Drawing for the job (mm, zero at the part's lowest x, y, z). Coordinates: 2 decimals unless noted, no trailing zeros. Use a Markdown table: item, result. Add a question column.
Q1. Wall check: L1, parallel to Z at x = 9.5, y = 1.8; L2, parallel to Y at x = 5, z = 2.25 (1 decimal); L3, parallel to Z at x = 15.25, y = 2.8. Give the ranges that are in metal, low to high. Write a range as from..to.
Q2. Slice it at A-A on x = 9.5. Count the separate pieces of the cut face and the enclosed holes in it.
Q3. Pin check, flat tips, straight feed: pin 1 Ø3 at (x, z) = (15.35, 9.5) entering from +Y (1 decimal); pin 2 Ø4.5 at (x, z) = (3.65, 9.5) entering from +Y; pin 3 Ø1 at (x, y) = (4, 1) entering from -Z; pin 4 Ø1 at (x, y) = (8, 0.5) entering from -Z. Stop position of each tip, or through.
Q4. Mould opens along Y. For the marked faces 1, 2 and 3 say: released by +Y, released by -Y, zero draft, split by the parting line, or undercut.
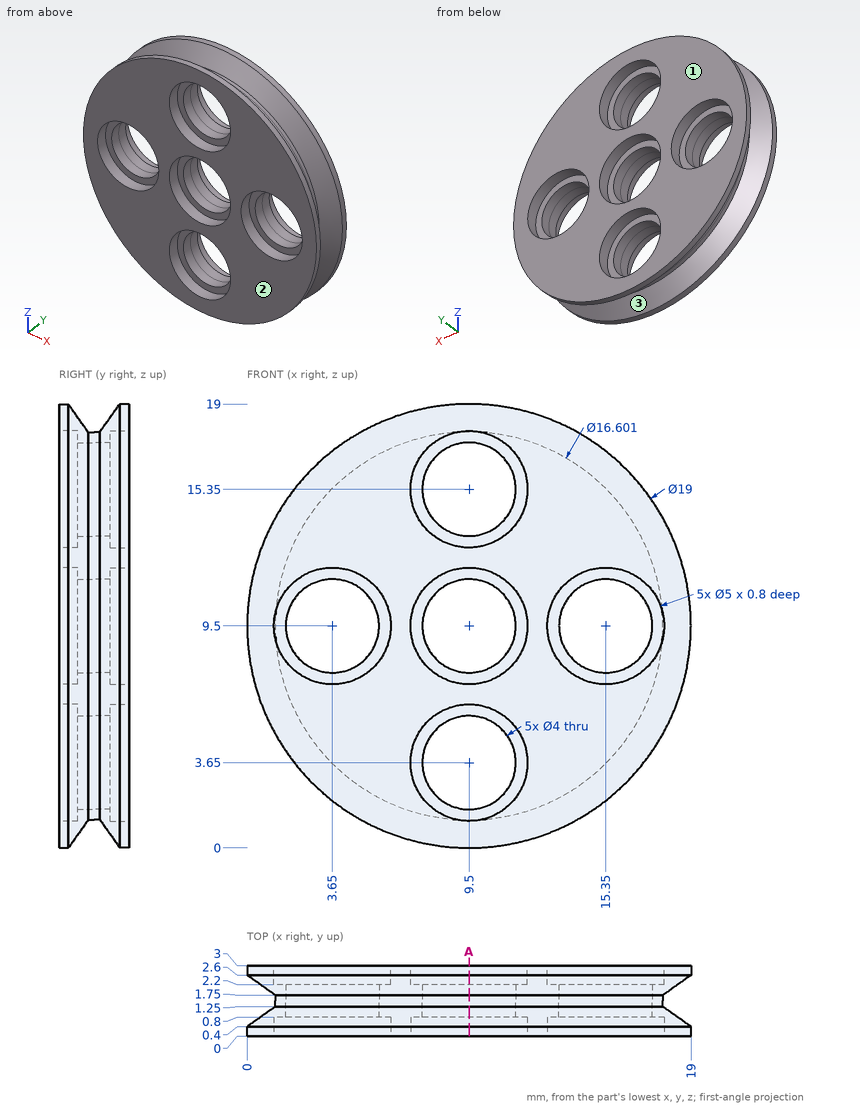
Recorded:
| question | item | result |
|---|---|---|
| 1 | L1 | 1.13..1.65, 5.65..7.5, 11.5..13.35, 17.35..17.87 |
| 1 | L2 | 0..1.1, 1.9..3 |
| 1 | L3 | 1.94..7, 12..17.06 |
| 2 | separate pieces | 4 |
| 2 | enclosed holes | 0 |
| 3 | pin 1 | through |
| 3 | pin 2 | y = 2.2 |
| 3 | pin 3 | z = 1.86 |
| 3 | pin 4 | z = 0.05 |
| 4 | face 1 | released by +Y |
| 4 | face 2 | released by -Y |
| 4 | face 3 | undercut |
